The drawing under review shows one solid part. Ordinate dimensions are in mm from its lowest x, y, z. A direction names the side the tool comes from. Coordinates: 2 decimals unless noted, no trailing zeros. Write each loop counter-clockwise with the first axis right and the second up, starting at its lowest first coordinate (ties: lowest second). Pieces come first, ordered by that corner, then holes.
Q1. Add section B-B, the plane z = 24.5. Give the boundary of the cut face in (x, y), plus the area to 3 significant figures.
Q2. Add section C-C, the plane x = 38.5. Give the boundary of the cut face in (y, z).
Q3. Machinability: for the marked faces 1, 2 and 3, which of the approach directions +Z, -Z, +X, -X, +Y, -Y give a long, thin tool a straight path to every point of the face, cutting with its end or side? Answer none if there is none.
Q4. Clearance check with flat-ended pins moving along their axes: pin 1 Ø5 at (y, z) = (111.5, 43) entering from +X; pin 2 Ø19.5 at (y, z) = (84, 33) entering from -X; pin 3 Ø5 at (x, y) = (52, 18) entering from +Z; pin 4 Ø12 at (x, z) = (57, 28) entering from -Y. State where each tip first meets the part, or that it passes through.
Q5. To check wall thickness, follow probe 1 along Z at (x, y) = (8, 51.5); probe 2 along X at (y, z) = (51, 25); probe 3 along X at (y, z) = (81.5, 11). State the ranges of each line that lie inside material, in increasing order.
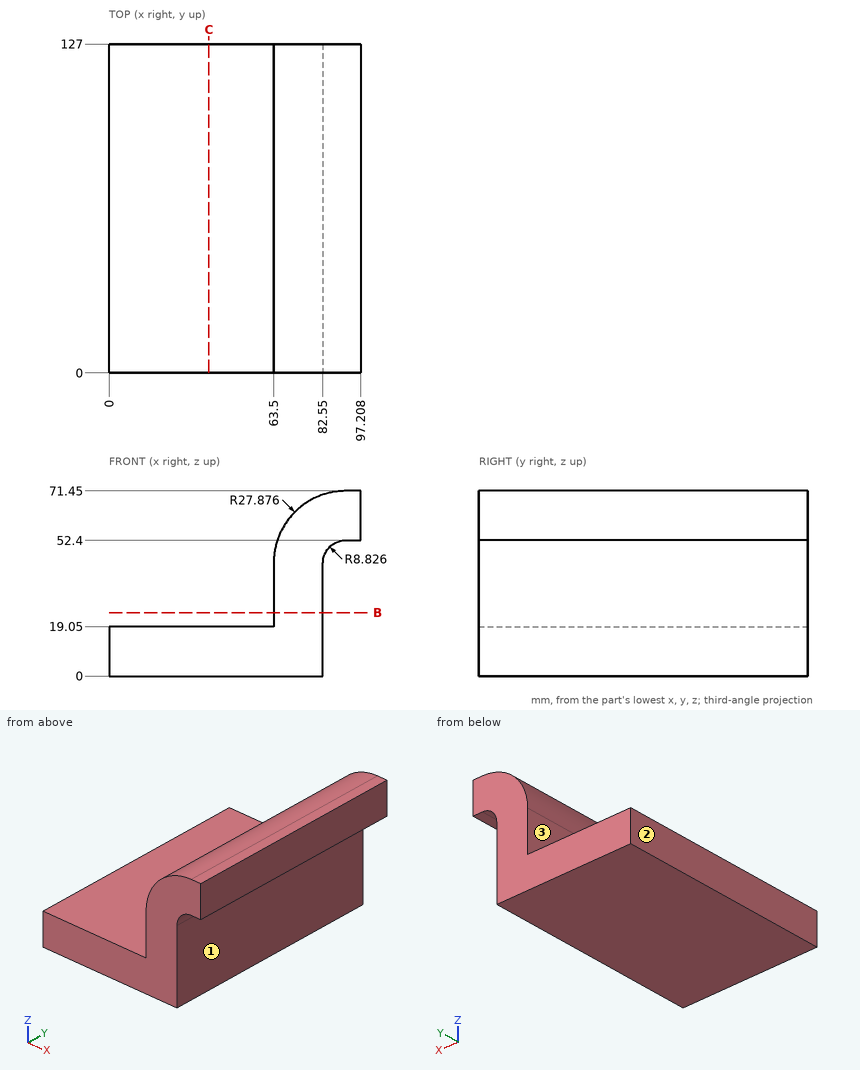
Here are the results:
1. outline: (63.5, 0) - (82.55, 0) - (82.55, 127) - (63.5, 127) - close
1. area: 2,420 mm2
2. outline: (0, 0) - (127, 0) - (127, 19.05) - (0, 19.05) - close
3. face 1: -Z, +X, +Y, -Y
3. face 2: +Z, -Z, -X, +Y, -Y
3. face 3: +Z, -X, +Y, -Y
4. pin 1: stops at x = 82.76
4. pin 2: stops at x = 63.5
4. pin 3: stops at z = 19.05
4. pin 4: passes through
5. probe 1: z = 0 to 19.05
5. probe 2: x = 63.5 to 82.55
5. probe 3: x = 0 to 82.55
